Could you check a few things on this model? Use its own coordinates, in mm. A direction names the side the tool comes from. Coordinates: 2 decimals unless noted, no trailing zeros. Order: outer loops, then holes, each group sorted by start corner. A loop starts at its lowest first (then second) coordinate and runs counter-clockwise, first axis right, second up. Notation, with made-up numbers: (53.5, 54) -> (77.5, 54) arc R33 cw to (77.5, 82) -> close; hole circle Ø4 at (-22, 37.25). An arc over 180 degrees is marked (long way). Use a Markdown table: item, result. Add a question column.
1) If I drill on L1, parallel to Y at x = 5.05, z = 4.15; L2, parallel to Z at x = 5.4, y = 2; L3, parallel to Z at x = 1.35, y = 1.9, over which ranges is the centre line in solid material (lowest first)? Write a range as [from, to].
2) If we section it at B-B (y = 2.45): Write out the boundary of the cut face in (x, z).
3) If we section it at C-C (x = 4.15): Write out the boundary of the cut face in (y, z).
4) If we section it at A-A (z = 2.65): Write out the boundary of the cut face in (x, y), plus the area to 4 significant figures.
5) Which directions (+Z, -Z, +X, -X, +Y, -Y) give clear straight access to the entire face, cutting with the end or side of a thin tool? Please do faces 1 (the flat face through (1, 3, 4)), 2 (the flat face through (4, 1, 4)), 3 (the flat face through (1, 2, 5)).
6) If we section it at D-D (z = 4.25): Write out the boundary of the cut face in (x, y), plus the area to 4 significant figures.
```python
from build123d import *

# Parameters (mm, degrees)
SKETCH1_W           = 6
SKETCH1_H           = 5
BOSS_EXTRUDE1_DEPTH = 5
CUT_EXTRUDE1_DEPTH  = 5
CUT_EXTRUDE2_DEPTH  = 2
CUT_EXTRUDE3_DEPTH  = 3


with BuildPart() as part:
    # Sketch1 → Boss-Extrude1 (new body)
    with BuildSketch(Plane.XY):
        with Locations((3, 2.5)):
            Rectangle(SKETCH1_W, SKETCH1_H)
    extrude(amount=BOSS_EXTRUDE1_DEPTH)

    # Sketch4 → Cut-Extrude1 (cut)
    with BuildSketch(Plane(origin=(0, 5, 0), x_dir=(1, 0, 0), z_dir=(0, 1, 0))):
        Polygon((0, -2), (2, 0), (0, 0), align=None)
    extrude(amount=-CUT_EXTRUDE1_DEPTH, mode=Mode.SUBTRACT)

    # Sketch5 → Cut-Extrude2 (cut)
    with BuildSketch(Plane(origin=(0, 5, 0), x_dir=(1, 0, 0), z_dir=(0, 1, 0))):
        Polygon((0, -2), (3, -5), (0, -5), align=None)
    extrude(amount=-CUT_EXTRUDE2_DEPTH, mode=Mode.SUBTRACT)

    # Sketch6 → Cut-Extrude3 (cut)
    with BuildSketch(Plane.XZ):
        Polygon((6, 5), (3, 5), (6, 2), align=None)
    extrude(amount=-CUT_EXTRUDE3_DEPTH, mode=Mode.SUBTRACT)


solid = part.part
```
Answer sheet:
| question | item | result |
|---|---|---|
| 1 | L1 | [3, 5] |
| 1 | L2 | [0, 2.6] |
| 1 | L3 | [0.65, 5] |
| 2 | outline | (0, 2) -> (2, 0) -> (6, 0) -> (6, 2) -> (3, 5) -> (0, 5) -> close |
| 3 | outline | (0, 0) -> (5, 0) -> (5, 5) -> (3, 5) -> (3, 3.85) -> (0, 3.85) -> close |
| 4 | outline | (0, 0) -> (5.35, 0) -> (5.35, 3) -> (6, 3) -> (6, 5) -> (0.65, 5) -> (0.65, 3) -> (0, 3) -> close |
| 4 | area | 26.75 mm2 |
| 5 | face 1 | +Z, -X, +Y |
| 5 | face 2 | +Z, +X, -Y |
| 5 | face 3 | +Z, +X, -X, +Y, -Y |
| 6 | outline | (0, 0) -> (3.75, 0) -> (3.75, 3) -> (6, 3) -> (6, 5) -> (2.25, 5) -> (2.25, 3) -> (0, 3) -> close |
| 6 | area | 18.75 mm2 |
